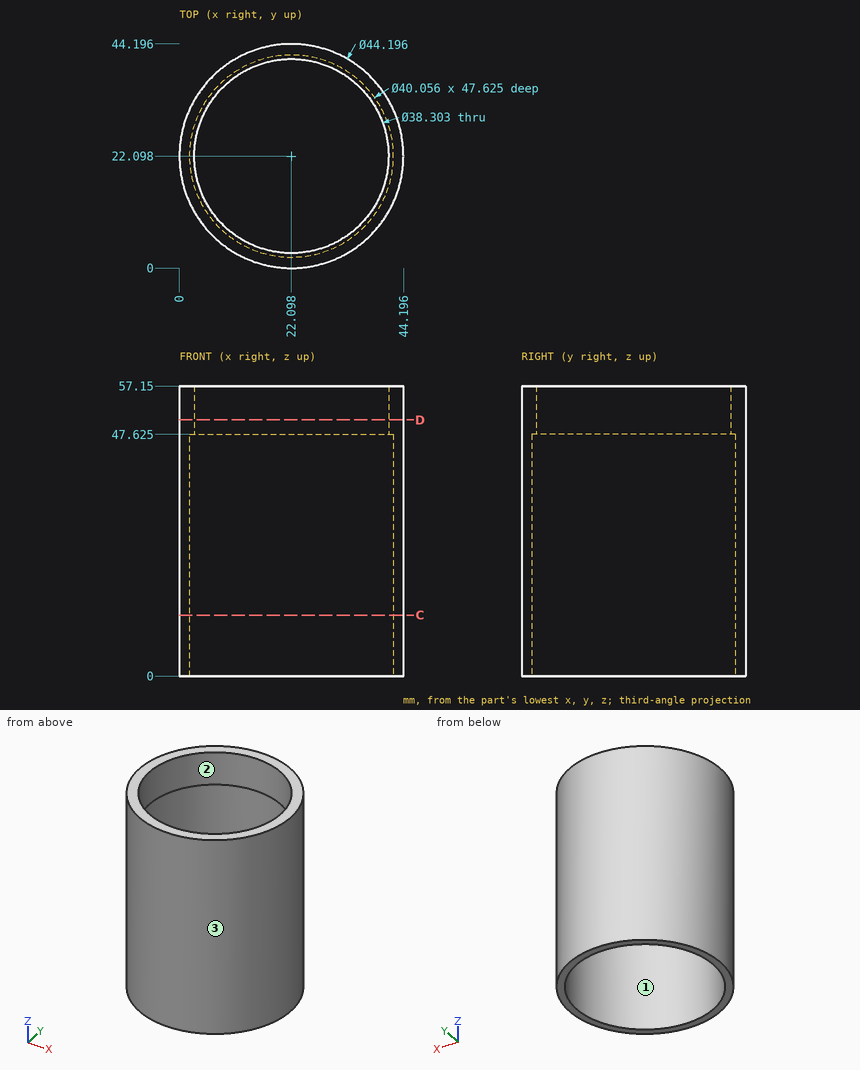
Part print with two shaded views. Sizes in mm from the minimum x, y, z corner. Round coordinates to 2 decimals unless told otherwise and drop trailing zeros. Loops run counter-clockwise (first coordinate to the right, second up) from the corner with the lowest first, then second, coordinate; pieces in that order, holes last.
Item 1: Saw through at D-D (z = 50.5). List the corners of the cut face in (x, y).
Item 2: Pin check, flat tips, straight feed: P1, Ø3, axis at y = 27, z = 32.5, coming from the +X side; P2, Ø3, axis at y = 18.5, z = 23, coming from the +X side; P3, Ø5, axis at x = 23.5, z = 42.5, coming from the +Y side. Stop position of each tip, or through.
Item 3: Saw through at C-C (z = 12). List the corners of the cut face in (x, y), then the cut area to 3 significant figures.
Item 4: Drill centre lines: line 1 along X through (y, z) = (22, 43); line 2 along X through (y, z) = (18.5, 14) (1 decimal); line 3 along Y through (x, z) = (12, 47). Where is each one in solid material? Low to high.
Item 5: Two-plate mould, pull along X, no slides. Class the marked faces 1, 2 and 3: released by +X, released by -X, zero draft, split by the parting line, or undercut.
Worked answers:
1. outline: circle Ø44.2 at (22.1, 22.1); hole circle Ø38.3 at (22.1, 22.1)
2. P1: stops at x = 43.93
2. P2: stops at x = 44.1
2. P3: stops at y = 44.2
3. outline: circle Ø44.2 at (22.1, 22.1); hole circle Ø40.06 at (22.1, 22.1)
3. area: 274 mm2
4. line 1: x = 0 to 2.07, 42.13 to 44.2
4. line 2: x = 0.3 to 2.4, 41.8 to 43.9
4. line 3: y = 2.44 to 4.8, 39.39 to 41.75
5. face 1: undercut
5. face 2: undercut
5. face 3: split by the parting line
